from build123d import *
from build123d.topology import SkipClean

# Parameters (mm, degrees)
BOSS_EXTRUDE1_DEPTH     = 3
BOSS_EXTRUDE2_START     = -67
SKETCH2_R               = 7.5
BOSS_EXTRUDE2_DEPTH     = 67
SKETCH4_W               = 8
SKETCH4_H               = 5
BOSS_EXTRUDE4_DEPTH     = 4
CUT_EXTRUDE1_DEPTH      = 72.994791478
CUT_EXTRUDE1_DEPTH_BACK = 72.994791478
SKETCH6_R               = 7.5
BOSS_EXTRUDE5_DEPTH     = 30


with BuildPart() as part:
    # Sketch1 → Boss-Extrude1 (new body)
    with BuildSketch(Plane(origin=(0, 0, 0), x_dir=(1, 0, 0), z_dir=(0, 1, 0))):
        with BuildLine():
            Line((-8.366600265, 1.5), (-7.348469228, 1.5))
            ThreePointArc((-7.348469228, 1.5), (-7.5, 0), (-7.348469228, -1.5))
            Line((-7.348469228, -1.5), (-8.366600265, -1.5))
            ThreePointArc((-8.366600265, -1.5), (0, -8.5), (8.366600265, -1.5))
            Line((8.366600265, -1.5), (7.348469228, -1.5))
            ThreePointArc((7.348469228, -1.5), (7.5, 0), (7.348469228, 1.5))
            Line((7.348469228, 1.5), (8.366600265, 1.5))
            ThreePointArc((8.366600265, 1.5), (0, 8.5), (-8.366600265, 1.5))
        make_face()
    extrude(amount=BOSS_EXTRUDE1_DEPTH)

    # Sketch2 → Boss-Extrude2 (add)
    with BuildSketch(Plane(origin=(0, 0, 0), x_dir=(1, 0, 0), z_dir=(0, 1, 0)).offset(BOSS_EXTRUDE2_START)):
        with Locations(Location((0, 0, 0), (0, 0, 168.463040967))):
            Circle(SKETCH2_R)
    extrude(amount=BOSS_EXTRUDE2_DEPTH)

    # Sketch4 → Boss-Extrude4 (add)
    with BuildSketch(Plane.XZ.offset(67)):
        Rectangle(SKETCH4_W, SKETCH4_H)
    extrude(amount=BOSS_EXTRUDE4_DEPTH)

    # Sketch5 → Cut-Extrude1 (cut, two sides: drawn at the far end of the back side and taken through both)
    with BuildSketch(Plane(origin=(0, 0, 0), x_dir=(0, 0, -1), z_dir=(1, 0, 0)).offset(-CUT_EXTRUDE1_DEPTH_BACK)):
        Polygon((-7.5, -51), (-3.5, -45), (-3.5, -44), (-7.5, -44), align=None)
        Polygon((7.5, -62), (3.5, -62), (3.5, -61), (7.5, -56), align=None)
    extrude(amount=CUT_EXTRUDE1_DEPTH + CUT_EXTRUDE1_DEPTH_BACK, mode=Mode.SUBTRACT)

    # Sketch6 → Boss-Extrude5 (add)
    with SkipClean():  # the faces are left unmerged after this step: merging them gives an invalid solid
        with BuildSketch(Plane(origin=(0, -67, 0), x_dir=(-1, 0, 0), z_dir=(0, -1, 0))):
            with Locations(Location((0, 0, 0), (0, 0, 11.536959033))):
                Circle(SKETCH6_R)
        extrude(amount=-BOSS_EXTRUDE5_DEPTH)


solid = part.part
The listing builds one solid part. Answer for the finished solid, in the listing's coordinates (mm). A direction names the side the tool comes from. Give positions to 0.01 mm unless a question says otherwise; leave off trailing zeros. Order: outer loops, then holes, each group sorted by start corner. A loop starts at its lowest first (then second) coordinate and runs counter-clockwise, first axis right, second up. Notation, with made-up numbers: (1.25, -14.5) -> (8.25, -14.5) arc R25 ccw to (8.25, 4.5) -> close; hole circle Ø6 at (-16, -30). An arc over 180 degrees is marked (long way). Put each result on its own line as item: value.
Item 1: For faces 1 (the face through (0, 0, 8)), 2 (the face through (-4, -69, 0)), 3 (the face through (-1, 0, -8)), 4 (the face through (0, -69, 2.5)), 5 (the face through (4, -69, 0)), determine the directions among +Z, -Z, +X, -X, +Y, -Y from which every point of the face is accessible in a straight line to the end or side of a thin tool.
Established:
face 1: +Z, -Y
face 2: +Z, -Z, -X, -Y
face 3: -Z, -Y
face 4: +Z, +X, -X, -Y
face 5: +Z, -Z, +X, -Y
Item 2: Straight lines are drawn through the part: line 1 (Y direction, x = -2.5, z = -7); line 2 (Z direction, x = -3.5, y = -57); line 3 (Y direction, x = 6.5, z = 4.5). For each, find the intervals that lie inside material, in ascending order.
Established:
line 1: y = -67 to 3
line 2: z = -6.63 to 6.63
line 3: y = 0 to 3
Item 3: A cutting plane is placed at D-D on x = 5.5. Give the vertices of the cut face in (y, z), plus the area to 3 significant figures.
Established:
outline: (-67, -5.1) -> (0, -5.1) -> (0, -6.48) -> (3, -6.48) -> (3, 6.48) -> (0, 6.48) -> (0, 5.1) -> (-67, 5.1) -> close
area: 722 mm^2
Item 4: A cutting plane is placed at B-B on z = 0. Give the vertices of the cut face in (x, y).
Established:
outline: (-7.5, -67) -> (-4, -67) -> (-4, -71) -> (4, -71) -> (4, -67) -> (7.5, -67) -> (7.5, 3) -> (-7.5, 3) -> close
Item 5: A cutting plane is placed at C-C on y = -14. Give the vertices of the cut face in (x, z), plus the area to 3 significant figures.
Established:
outline: circle Ø15 at (0, 0)
area: 177 mm^2
Item 6: A cutting plane is placed at A-A on x = 0. Give the vertices of the cut face in (y, z).
Established:
outline: (-71, -2.5) -> (-67, -2.5) -> (-67, -7.5) -> (0, -7.5) -> (0, -8.5) -> (3, -8.5) -> (3, 8.5) -> (0, 8.5) -> (0, 7.5) -> (-67, 7.5) -> (-67, 2.5) -> (-71, 2.5) -> close
Item 7: Given P1, Ø0.8, axis at x = 8, y = 1.5, coming from the -Z side; P2, Ø4, axis at y = -9, z = 3, coming from the -X side; P3, Ø0.8, axis at x = 8, y = 2, coming from the +Z side, each flat-ended and moving along its own axis, determine where each tip first touches the part or whether it passes through.
Established:
P1: stops at z = -3.81
P2: stops at x = -7.43
P3: stops at z = 3.81
